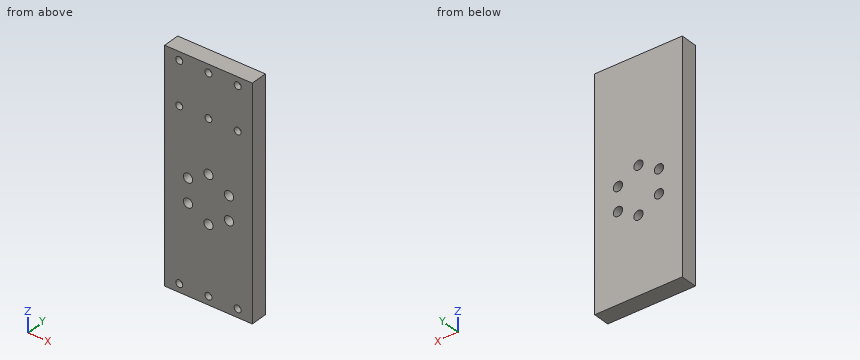
from build123d import *

# Parameters (mm, degrees)
SKETCH1_W                 = 50
SKETCH1_H                 = 130
BOSS_EXTRUDE1_DEPTH       = 9.525
F_4_0MM_DOWEL_HOLE1_D     = 4
F_4_0MM_DOWEL_HOLE1_DEPTH = 3.2
F_4_0MM_DOWEL_HOLE1_TIP   = 1.201721238
M5_CLEARANCE_HOLE1_D      = 5.3


with BuildPart() as part:
    # Sketch1 → Boss-Extrude1 (new body)
    with BuildSketch(Plane(origin=(0, 0, 0), x_dir=(1, 0, 0), z_dir=(0, 1, 0))):
        Rectangle(SKETCH1_W, SKETCH1_H)
    extrude(amount=BOSS_EXTRUDE1_DEPTH)

    # Ø4.0mm Dowel Hole1
    with Locations(Plane.XZ):
        with Locations((-16.67, 60.2375), (-16.67, -60.2375), (0, -60.2375), (16.67, -60.2375), (16.67, 35.7), (0, 35.7), (-16.67, 35.7), (16.67, 60.2375), (0, 60.2375)):
            Hole(F_4_0MM_DOWEL_HOLE1_D / 2, depth=F_4_0MM_DOWEL_HOLE1_DEPTH)
            with Locations((0, 0, -(F_4_0MM_DOWEL_HOLE1_DEPTH + F_4_0MM_DOWEL_HOLE1_TIP / 2))):  # 118° drill point
                Cone(0, F_4_0MM_DOWEL_HOLE1_D / 2, F_4_0MM_DOWEL_HOLE1_TIP, mode=Mode.SUBTRACT)

    # M5 Clearance Hole1 (through all)
    with Locations(Plane(origin=(0, 9.525, 0), x_dir=(1, 0, 0), z_dir=(0, 1, 0))):
        with Locations((-11.691342951, 14.72), (0, 21.47), (11.691342951, 14.72), (11.691342951, 1.22), (0, -5.53), (-11.691342951, 1.22)):
            Hole(M5_CLEARANCE_HOLE1_D / 2)


solid = part.part
Verification items for the finished model (mm, model axes). Give positions to 0.01 mm unless a question says otherwise; leave off trailing zeros. Loops run counter-clockwise (first coordinate to the right, second up) from the corner with the lowest first, then second, coordinate; pieces in that order, holes last.
1) Sectioned sample at A-A, the plane z = 5.53. Enter the section's corners in (x, y) (3 decimals), then the cut area to 3 significant figures.
2) Depth check by flat-ended pin: pin 1 Ø8.5 at (x, z) = (0, 5.53) entering from -Y; pin 2 Ø3.5 at (x, z) = (16.67, 35.7) entering from -Y. Enter the tip coordinate at first touch or a pass-through.
3) Sectioned sample at C-C, the plane x = 11.5. Enter the section's corners in (y, z) (3 decimals), then the cut area to 3 significant figures.
4) Sectioned sample at B-B, the plane y = 8. Enter the section's corners in (x, z), then the cut area to 3 significant figures.
5) Thickness scan on line 1 along Z through (x, y) = (0, 2.15); line 2 along Z through (x, y) = (16.67, 1.1); line 3 along Z through (x, y) = (0, 6.75). Record the ranges inside material, lowest first.
Answers:
1. outline: (-25, 0) - (-2.65, 0) - (-2.65, 9.525) - (-25, 9.525) - close; (2.65, 0) - (25, 0) - (25, 9.525) - (2.65, 9.525) - close
1. area: 426 mm2
2. pin 1: stops at y = 0
2. pin 2: stops at y = 3.35
3. outline: (0, -65) - (9.525, -65) - (9.525, -17.363) - (0, -17.363) - close; (0, -12.077) - (9.525, -12.077) - (9.525, -3.863) - (0, -3.863) - close; (0, 1.423) - (9.525, 1.423) - (9.525, 65) - (0, 65) - close
3. area: 1,140 mm2
4. outline: (-25, -65) - (25, -65) - (25, 65) - (-25, 65) - close; hole circle Ø5.3 at (-11.69, -14.72); hole circle Ø5.3 at (-11.69, -1.22); hole circle Ø5.3 at (0, -21.47); hole circle Ø5.3 at (0, 5.53); hole circle Ø5.3 at (11.69, -14.72); hole circle Ø5.3 at (11.69, -1.22)
4. area: 6,370 mm2
5. line 1: z = -65 to -62.24, -58.24 to -24.12, -18.82 to 2.88, 8.18 to 33.7, 37.7 to 58.24, 62.24 to 65
5. line 2: z = -65 to -62.24, -58.24 to 33.7, 37.7 to 58.24, 62.24 to 65
5. line 3: z = -65 to -24.12, -18.82 to 2.88, 8.18 to 65
